Read the model definition and answer for the solid it produces. Units are mm, in the model's axes. Coordinates: 2 decimals unless noted, no trailing zeros. Order: outer loops, then holes, each group sorted by start corner. A loop starts at its lowest first (then second) coordinate and runs counter-clockwise, first axis right, second up. Notation, with made-up numbers: (-16.75, 30) -> (20.25, 30) arc R24 ccw to (20.25, 55) -> close; hole circle Ø11 at (58, 30.5). An arc over 180 degrees is marked (long way). Use CSV: the item, a comma, the result in double quotes.
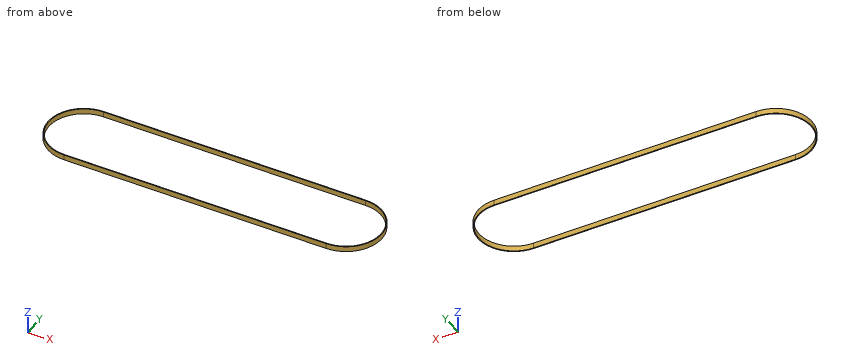
```python
from build123d import *

# Parameters (mm, degrees)
PAD_DEPTH = 6


with BuildPart() as part:
    # Sketch → Pad (new body)
    with BuildSketch(Plane.XY):
        with BuildLine():
            ThreePointArc((0, 41), (-41, 0), (0, -41))
            Line((300.000005, -41), (0, -41))
            ThreePointArc((300.000005, -41), (341, 0), (300.000005, 41))
            Line((0, 41), (300.000005, 41))
        make_face()
        with BuildLine():
            ThreePointArc((0, 40), (-40, 0), (0, -40))
            Line((0, -40), (300.000002, -40))
            ThreePointArc((300.000002, -40), (340, 0), (300.000001, 40))
            Line((0, 40), (300.000001, 40))
        make_face(mode=Mode.SUBTRACT)
    extrude(amount=PAD_DEPTH)


solid = part.part
```
Item 1: Find section B-B, the plane z = 1. Give the vertices of the cut face in (x, y).
Return value:
outline,"(0, -41) -> (300, -41) arc R41 ccw to (300, 41) -> (0, 41) arc R41 ccw to start; hole (0, -40) -> (300, -40) arc R40 ccw to (300, 40) -> (0, 40) arc R40 ccw to start"
Item 2: Each of these flat-tipped pins is pushed along its axis until it touches: P1, Ø1, axis at y = -9, z = 4.5, coming from the +X side; P2, Ø1.5, axis at y = -17, z = 3.5, coming from the -X side. Where does it stop, or does it pass through?
Return value:
P1,"stops at x = 340.11"
P2,"stops at x = -37.64"
Item 3: Straight lines are drawn through the part: line 1 along Y through (x, z) = (114, 1.8); line 2 along X through (y, z) = (-1, 0.55); line 3 along X through (y, z) = (-22, 2.9). For each, find the intervals that lie inside material, in ascending order.
Return value:
line 1,"y = -41 to -40, 40 to 41"
line 2,"x = -40.99 to -39.99, 339.99 to 340.99"
line 3,"x = -34.6 to -33.41, 333.41 to 334.6"
Item 4: Find section C-C, the plane x = 50.5. Give the vertices of the cut face in (y, z).
Return value:
outline,"(-41, 0) -> (-40, 0) -> (-40, 6) -> (-41, 6) -> close; (40, 0) -> (41, 0) -> (41, 6) -> (40, 6) -> close"
Item 5: Find section A-A, the plane y = 0. Give the vertices of the cut face in (x, z).
Return value:
outline,"(-41, 0) -> (-40, 0) -> (-40, 6) -> (-41, 6) -> close; (340, 0) -> (341, 0) -> (341, 6) -> (340, 6) -> close"
